from build123d import *

# Parameters (mm, degrees)
SKETCH2_W           = 58
SKETCH2_H           = 20.5
SKETCH2_R           = 8
SKETCH2_R_2         = 1.55
BOSS_EXTRUDE1_DEPTH = 2
SKETCH3_W           = 8.35
SKETCH3_H           = 8.75
SKETCH3_R           = 1.55
BOSS_EXTRUDE2_DEPTH = 9
SKETCH4_W           = 5
SKETCH4_H           = 20.5
BOSS_EXTRUDE3_DEPTH = 2


with BuildPart() as part:
    # Sketch2 → Boss-Extrude1 (new body)
    with BuildSketch(Plane(origin=(0, 0, 0), x_dir=(1, 0, 0), z_dir=(0, 1, 0))):
        Rectangle(SKETCH2_W, SKETCH2_H)
        with Locations((-9.65, 0)):
            Circle(SKETCH2_R, mode=Mode.SUBTRACT)
        with Locations((-24.5, 5)):
            Circle(SKETCH2_R_2, mode=Mode.SUBTRACT)
        with Locations((-24.5, -5)):
            Circle(SKETCH2_R_2, mode=Mode.SUBTRACT)
        with Locations((24.5, 5)):
            Circle(SKETCH2_R_2, mode=Mode.SUBTRACT)
        with Locations((24.5, -5)):
            Circle(SKETCH2_R_2, mode=Mode.SUBTRACT)
        with Locations((9.65, 0)):
            Circle(SKETCH2_R, mode=Mode.SUBTRACT)
    extrude(amount=BOSS_EXTRUDE1_DEPTH)

    # Sketch3 → Boss-Extrude2 (add)
    with BuildSketch(Plane.XZ):
        with Locations((-24.825, 5.875)):
            Rectangle(SKETCH3_W, SKETCH3_H)
        with Locations((-24.5, 5)):
            Circle(SKETCH3_R, mode=Mode.SUBTRACT)
        with Locations((-24.825, -5.875)):
            Rectangle(SKETCH3_W, SKETCH3_H)
        with Locations((-24.5, -5)):
            Circle(SKETCH3_R, mode=Mode.SUBTRACT)
        with Locations((24.825, 5.875)):
            Rectangle(SKETCH3_W, SKETCH3_H)
        with Locations((24.5, 5)):
            Circle(SKETCH3_R, mode=Mode.SUBTRACT)
        with Locations((24.825, -5.875)):
            Rectangle(SKETCH3_W, SKETCH3_H)
        with Locations((24.5, -5)):
            Circle(SKETCH3_R, mode=Mode.SUBTRACT)
    extrude(amount=BOSS_EXTRUDE2_DEPTH)

    # Sketch4 → Boss-Extrude3 (add)
    with BuildSketch(Plane(origin=(0, 2, 0), x_dir=(1, 0, 0), z_dir=(0, 1, 0))):
        with Locations((-31.5, 0)):
            Rectangle(SKETCH4_W, SKETCH4_H)
        with Locations((31.5, 0)):
            Rectangle(SKETCH4_W, SKETCH4_H)
    extrude(amount=-BOSS_EXTRUDE3_DEPTH)


solid = part.part
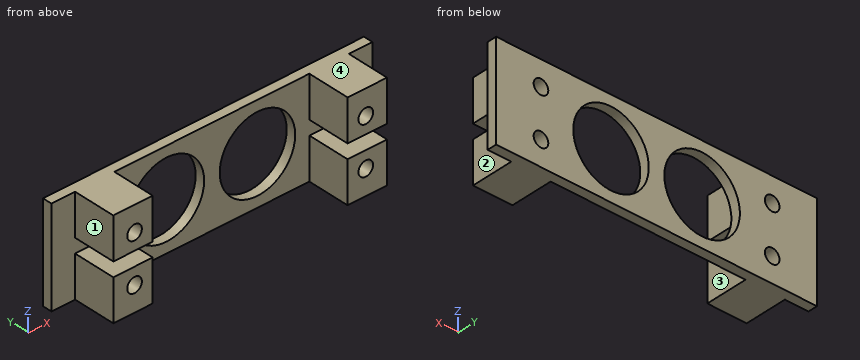
CAD build for the part. Positions are in the model's coordinates, mm. Face numbers are marked on the shaded views. A direction names the side the tool comes from. Coordinates: 2 decimals unless noted, no trailing zeros. Order: outer loops, then holes, each group sorted by start corner. A loop starts at its lowest first (then second) coordinate and runs counter-clockwise, first axis right, second up. Notation, with made-up numbers: (30.5, 69.25) -> (60.5, 69.25) arc R24 cw to (60.5, 105.25) -> close; hole circle Ø10 at (35.5, 24.5). An arc over 180 degrees is marked (long way). Answer in a Markdown table with one row per item.
1) Which spindle directions (+Z, -Z, +X, -X, +Y, -Y) get a long thin tool onto all of the face, cutting with end or side? Do the marked faces 1, 2, 3 and 4. Say none if no direction does.
Check values:
| item | result |
|---|---|
| face 1 | +Z, -Z, -X, -Y |
| face 2 | +Z, -Z, +X, -Y |
| face 3 | +Z, -Z, -Y |
| face 4 | +Z, +X, -X, +Y, -Y |
2) Band-saw the part on D-D (x = 9.65). List the corners of the cut face in (y, z), and give its area (3 significant figures).
Check values:
| item | result |
|---|---|
| outline | (0, -10.25) -> (2, -10.25) -> (2, -8) -> (0, -8) -> close; (0, 8) -> (2, 8) -> (2, 10.25) -> (0, 10.25) -> close |
| area | 9.00 mm2 |
3) Band-saw the part on C-C (x = 24.5). List the corners of the cut face in (y, z).
Check values:
| item | result |
|---|---|
| outline | (-9, -10.25) -> (2, -10.25) -> (2, -6.55) -> (-9, -6.55) -> close; (-9, -3.45) -> (2, -3.45) -> (2, 3.45) -> (-9, 3.45) -> (-9, 1.5) -> (0, 1.5) -> (0, -1.5) -> (-9, -1.5) -> close; (-9, 6.55) -> (2, 6.55) -> (2, 10.25) -> (-9, 10.25) -> close |
4) Drill centre lines: line 1 (X direction, y = -4, z = -5); line 2 (Z direction, x = 24.5, y = -0.25); line 3 (X direction, y = -3, z = -8.75). Where is each one in solid material? Low to high.
Check values:
| item | result |
|---|---|
| line 1 | -29 to -26.05, -22.95 to -20.65, 20.65 to 22.95, 26.05 to 29 |
| line 2 | -10.25 to -6.55, -3.45 to -1.5, 1.5 to 3.45, 6.55 to 10.25 |
| line 3 | -29 to -20.65, 20.65 to 29 |
5) Band-saw the part on B-B (y = -6). List the corners of the cut face in (x, z).
Check values:
| item | result |
|---|---|
| outline | (-29, -10.25) -> (-20.65, -10.25) -> (-20.65, -1.5) -> (-29, -1.5) -> close; (-29, 1.5) -> (-20.65, 1.5) -> (-20.65, 10.25) -> (-29, 10.25) -> close; (20.65, -10.25) -> (29, -10.25) -> (29, -1.5) -> (20.65, -1.5) -> close; (20.65, 1.5) -> (29, 1.5) -> (29, 10.25) -> (20.65, 10.25) -> close; hole circle Ø3.1 at (-24.5, -5); hole circle Ø3.1 at (-24.5, 5); hole circle Ø3.1 at (24.5, -5); hole circle Ø3.1 at (24.5, 5) |
6) Band-saw the part on A-A (z = 0). List the corners of the cut face in (x, y), and give its area (3 significant figures).
Check values:
| item | result |
|---|---|
| outline | (-34, 0) -> (-17.65, 0) -> (-17.65, 2) -> (-34, 2) -> close; (-1.65, 0) -> (1.65, 0) -> (1.65, 2) -> (-1.65, 2) -> close; (17.65, 0) -> (34, 0) -> (34, 2) -> (17.65, 2) -> close |
| area | 72.0 mm2 |
7) Flat gauge pins, fed straight in: P1, Ø4.5, axis at y = -6, z = -5.5, coming from the -X side; P2, Ø2, axis at y = -6.5, z = 1, coming from the +X side. Where does each tip first touch, or does it go through?
Check values:
| item | result |
|---|---|
| P1 | x = -29 |
| P2 | x = 29 |
